Can you work these out from the model? Positions are in its coordinate system, mm. A direction names the side the tool comes from. Give positions to 0.01 mm unless a question says otherwise; leave off trailing zeros. Loops run counter-clockwise (first coordinate to the right, second up) from the corner with the lowest first, then second, coordinate; pieces in that order, holes last.
from build123d import *

# Parameters (mm, degrees)
F0_R           = 76.2
F1_DEPTH       = 25.4
F4_D           = 6.5278
F4_DEPTH       = 76.2
F4_CBORE_D     = 9.525
F4_CBORE_DEPTH = 25.4


with BuildPart() as f1:
    # F0 (on Right) → F1 (new body, symmetric)
    with BuildSketch(Plane.YZ):
        Circle(F0_R)
        with BuildLine():
            ThreePointArc((3.9624, 17.007007), (0, -17.4625), (-3.9624, 17.007007))
            Line((-3.9624, 17.007007), (-3.9624, 21.5265))
            Line((-3.9624, 21.5265), (3.9624, 21.5265))
            Line((3.9624, 21.5265), (3.9624, 17.007007))
        make_face(mode=Mode.SUBTRACT)
    extrude(amount=F1_DEPTH, both=True)

    # F4
    with Locations(Plane.XY.offset(76.2)):
        with Locations((0, 0)):
            CounterBoreHole(F4_D / 2, F4_CBORE_D / 2, F4_CBORE_DEPTH, depth=F4_DEPTH)


solid = f1.part
(1) Suppose I cut it at A-A on y = 0. List the corners of the cut face in (x, z) for me, plus the area to 3 significant figures.
Returned:
outline: (-25.4, -76.2) - (25.4, -76.2) - (25.4, -17.46) - (-25.4, -17.46) - close; (-25.4, 21.53) - (-3.26, 21.53) - (-3.26, 50.8) - (-4.76, 50.8) - (-4.76, 76.2) - (-25.4, 76.2) - close; (3.26, 21.53) - (25.4, 21.53) - (25.4, 76.2) - (4.76, 76.2) - (4.76, 50.8) - (3.26, 50.8) - close
area: 5,330 mm2
(2) Suppose I cut it at C-C on x = -18. List the corners of the cut face in (y, z) for me (1 decimal), plus the area to 3 significant figures.
Returned:
outline: circle Ø152.4 at (0, 0); hole (-4, 17) arc R17.5 ccw (long way) to (4, 17) - (4, 21.5) - (-4, 21.5) - close
area: 17,300 mm2
(3) Suppose I cut it at B-B on z = 0. List the corners of the cut face in (x, y) for me.
Returned:
outline: (-25.4, -76.2) - (25.4, -76.2) - (25.4, -17.46) - (-25.4, -17.46) - close; (-25.4, 17.46) - (25.4, 17.46) - (25.4, 76.2) - (-25.4, 76.2) - close
(4) Thinking about a two-plate mould opening in X: for faces 1 (the flat face through (25.4, -18, 1)), 2 (the flat face through (0, -3.962, 19)), 3 (the cylindrical face through (-3.78, -2.9, 63.68)), 4 (the flat face through (-25.4, -18, 1)), which applies, pulls with the +X half, pulls with the -X half, needs draft (parallel to the pull), parting line crosses it, or undercut?
Returned:
face 1: pulls with the +X half
face 2: needs draft
face 3: undercut
face 4: pulls with the -X half
(5) Will these pins go through, and if not, where does the flat tip stop? P1, Ø1.5, axis at x = -13, y = -44.5, coming from the +Z side; P2, Ø10, axis at x = -4.5, y = 16.5, coming from the -Z side; P3, Ø10, axis at x = -8.5, y = -51.5, coming from the -Z side.
Returned:
P1: stops at z = 62.39
P2: stops at z = -75.33
P3: stops at z = -60.37
(6) Please list where these lines run through material, in increasing order: probe 1 along X at (y, z) = (0, 66); probe 2 along Z at (x, y) = (15, 0); probe 3 along Z at (x, y) = (-6, 12.5).
Returned:
probe 1: x = -25.4 to -4.76, 4.76 to 25.4
probe 2: z = -76.2 to -17.46, 21.53 to 76.2
probe 3: z = -75.17 to -12.19, 12.19 to 75.17
(7) Which directions (+Z, -Z, +X, -X, +Y, -Y) give clear straight access to the entire face, cutting with the end or side of a thin tool? Please do faces 5 (the flat face through (0.4, 3.5, 21.526)), 6 (the cylindrical face through (0.708, -3.186, 35.958)).
Returned:
face 5: +X, -X
face 6: +Z
(8) Suppose I cut it at D-D on x = 0. List the corners of the cut face in (y, z) for me (1 decimal), plus the area to 3 significant figures.
Returned:
outline: (-4.8, 50.8) - (-4.8, 76.1) arc R76.2 ccw (long way) to (4.8, 76.1) - (4.8, 50.8) - (3.3, 50.8) - (3.3, 21.5) - (4, 21.5) - (4, 17) arc R17.5 cw (long way) to (-4, 17) - (-4, 21.5) - (-3.3, 21.5) - (-3.3, 50.8) - close
area: 16,800 mm2
